```python
from build123d import *
from build123d.topology import SkipClean

# Parameters (mm, degrees)
BOSS_EXTRUDE1_DEPTH           = 3
BOSS_EXTRUDE2_START           = -1.75
SKETCH1_3_R                   = 11
BOSS_EXTRUDE2_DEPTH           = 1.75
SKETCH2_R                     = 1.75
CUT_EXTRUDE1_DEPTH            = 4.75
SKETCH2_3_R                   = 3
CUT_EXTRUDE2_DEPTH            = 1.75
SKETCH1_6_W                   = 11
SKETCH1_6_H                   = 6
BOSS_EXTRUDE3_DEPTH           = 5
SKETCH3_R                     = 1.35
CUT_EXTRUDE3_DEPTH            = 8
LPATTERN1_COUNT               = 2
LPATTERN1_PITCH               = 8
LPATTERN1_COL_COUNT           = 2
LPATTERN1_COL_PITCH           = 8
BODY_MOVE_COPY1_START         = -3
BODY_MOVE_COPY1_OUTLINE_R     = 3
BODY_MOVE_COPY1_DEPTH         = 3
BODY_MOVE_COPY1_START_2       = 3
BODY_MOVE_COPY1_2_OUTLINE_W   = 22
BODY_MOVE_COPY1_2_OUTLINE_H   = 6
BODY_MOVE_COPY1_2_OUTLINE_R   = 1.35
BODY_MOVE_COPY1_2_DEPTH       = 2
BODY_MOVE_COPY1_START_3       = 1.25
BODY_MOVE_COPY1_3_OUTLINE_R   = 3
BODY_MOVE_COPY1_3_OUTLINE_R_2 = 1.75
BODY_MOVE_COPY1_3_DEPTH       = 0.5
BODY_MOVE_COPY1_4_DEPTH       = 3
BODY_MOVE_COPY1_START_4       = 1.75
BODY_MOVE_COPY1_5_OUTLINE_R   = 11
BODY_MOVE_COPY1_5_OUTLINE_R_2 = 3
BODY_MOVE_COPY1_5_DEPTH       = 1.25
BODY_MOVE_COPY1_START_5       = -5
BODY_MOVE_COPY1_6_OUTLINE_W   = 22
BODY_MOVE_COPY1_6_OUTLINE_H   = 6
BODY_MOVE_COPY1_6_OUTLINE_R   = 1.35
BODY_MOVE_COPY1_6_DEPTH       = 2
BODY_MOVE_COPY1_START_6       = -1.75
BODY_MOVE_COPY1_7_OUTLINE_R   = 3
BODY_MOVE_COPY1_7_OUTLINE_R_2 = 1.75
BODY_MOVE_COPY1_7_DEPTH       = 0.5


# Read off the part's stored shape, not the designer's step: Body-Move/Copy1
with BuildPart() as part:
    # Sketch1 → Boss-Extrude1 (new body)
    with BuildSketch(Plane.XY):
        with BuildLine():
            Line((-11, 30), (-11, -30))
            Line((-11, -30), (11, -30))
            Line((11, -30), (11, 30))
            ThreePointArc((11, 30), (0, 41), (-11, 30))
        make_face()
        with BuildLine():
            Line((5, -23), (-5, -23))
            Line((-5, -23), (-5, 19.643842411))
            ThreePointArc((-5, 19.643842411), (0, 18.5), (5, 19.643842411))
            Line((5, 19.643842411), (5, -23))
        make_face(mode=Mode.SUBTRACT)
    extrude(amount=BOSS_EXTRUDE1_DEPTH)

    # Sketch1<3> → Boss-Extrude2 (add)
    with BuildSketch(Plane.XY.offset(BOSS_EXTRUDE2_START)):
        with Locations((0, 30)):
            Circle(SKETCH1_3_R)
    extrude(amount=BOSS_EXTRUDE2_DEPTH)

    # Sketch2 → Cut-Extrude1 (cut)
    with BuildSketch(Plane.XY.offset(3)):
        with Locations((0, 30)):
            Circle(SKETCH2_R)
    extrude(amount=-CUT_EXTRUDE1_DEPTH, mode=Mode.SUBTRACT)

    # Sketch2<3> → Cut-Extrude2 (cut)
    with BuildSketch(Plane.XY.offset(3)):
        with Locations((0, 30)):
            Circle(SKETCH2_3_R)
    extrude(amount=-CUT_EXTRUDE2_DEPTH, mode=Mode.SUBTRACT)

    # Sketch1<6> → Boss-Extrude3 (add)
    with BuildSketch(Plane.XY):
        with Locations((5.5, -27)):
            Rectangle(SKETCH1_6_W, SKETCH1_6_H)
        with Locations((-5.5, -27)):
            Rectangle(SKETCH1_6_W, SKETCH1_6_H)
    extrude(amount=-BOSS_EXTRUDE3_DEPTH)

    # Sketch3 → Cut-Extrude3 (cut)
    with BuildSketch(Plane.XY.offset(3)):
        with Locations((0, -26.6)):
            Circle(SKETCH3_R)
    cut_extrude3 = extrude(amount=-CUT_EXTRUDE3_DEPTH, mode=Mode.SUBTRACT)

    # LPattern1: Cut-Extrude3 ×2
    with Locations(*[(i * LPATTERN1_PITCH, 0, 0) for i in range(1, LPATTERN1_COUNT)]):
        add(cut_extrude3, mode=Mode.SUBTRACT)

    # LPattern1 col: Cut-Extrude3 ×2
    with Locations(*[(-i * LPATTERN1_COL_PITCH, 0, 0) for i in range(1, LPATTERN1_COL_COUNT)]):
        add(cut_extrude3, mode=Mode.SUBTRACT)

    # Body-Move/Copy1 outline → Body-Move/Copy1 (add)
    with BuildSketch(Plane.XY.offset(BODY_MOVE_COPY1_START)):
        with BuildLine():
            Line((-11, 30), (-11, -24))
            Line((-11, -24), (11, -24))
            Line((11, -24), (11, 30))
            ThreePointArc((11, 30), (0, 41), (-11, 30))
        make_face()
        with BuildLine():
            Line((-5, -23), (-5, 19.643842411))
            ThreePointArc((-5, 19.643842411), (0, 18.5), (5, 19.643842411))
            Line((5, 19.643842411), (5, -23))
            Line((5, -23), (-5, -23))
        make_face(mode=Mode.SUBTRACT)
        with Locations((0, 30)):
            Circle(BODY_MOVE_COPY1_OUTLINE_R, mode=Mode.SUBTRACT)
    extrude(amount=BODY_MOVE_COPY1_DEPTH)

    # Body-Move_Copy1 2 outline → Body-Move_Copy1 2 (add)
    with BuildSketch(Plane.XY.offset(BODY_MOVE_COPY1_START_2)):
        with Locations((0, -27)):
            Rectangle(BODY_MOVE_COPY1_2_OUTLINE_W, BODY_MOVE_COPY1_2_OUTLINE_H)
        with Locations((-8, -26.6)):
            Circle(BODY_MOVE_COPY1_2_OUTLINE_R, mode=Mode.SUBTRACT)
        with Locations((0, -26.6)):
            Circle(BODY_MOVE_COPY1_2_OUTLINE_R, mode=Mode.SUBTRACT)
        with Locations((8, -26.6)):
            Circle(BODY_MOVE_COPY1_2_OUTLINE_R, mode=Mode.SUBTRACT)
    extrude(amount=BODY_MOVE_COPY1_2_DEPTH)

    # Body-Move_Copy1 3 outline → Body-Move_Copy1 3 (add)
    with BuildSketch(Plane.XY.offset(BODY_MOVE_COPY1_START_3)):
        with Locations((0, 30)):
            Circle(BODY_MOVE_COPY1_3_OUTLINE_R)
        with Locations((0, 30)):
            Circle(BODY_MOVE_COPY1_3_OUTLINE_R_2, mode=Mode.SUBTRACT)
    extrude(amount=BODY_MOVE_COPY1_3_DEPTH)

    # Body-Move_Copy1 4 outline → Body-Move_Copy1 4 (cut)
    with SkipClean():  # the faces are left unmerged after this step: merging them gives an invalid solid
        with BuildSketch(Plane.XY):
            with BuildLine():
                Line((-11, 30), (-11, -24))
                Line((-11, -24), (11, -24))
                Line((11, -24), (11, 30))
                ThreePointArc((11, 30), (0, 19), (-11, 30))
            make_face()
            with BuildLine():
                Line((-5, -23), (-5, 19.643842411))
                ThreePointArc((-5, 19.643842411), (0, 18.5), (5, 19.643842411))
                Line((5, 19.643842411), (5, -23))
                Line((5, -23), (-5, -23))
            make_face(mode=Mode.SUBTRACT)
        extrude(amount=BODY_MOVE_COPY1_4_DEPTH, mode=Mode.SUBTRACT)

    # Body-Move_Copy1 5 outline → Body-Move_Copy1 5 (cut)
    with BuildSketch(Plane.XY.offset(BODY_MOVE_COPY1_START_4)):
        with Locations((0, 30)):
            Circle(BODY_MOVE_COPY1_5_OUTLINE_R)
        with Locations((0, 30)):
            Circle(BODY_MOVE_COPY1_5_OUTLINE_R_2, mode=Mode.SUBTRACT)
    extrude(amount=BODY_MOVE_COPY1_5_DEPTH, mode=Mode.SUBTRACT)

    # Body-Move_Copy1 6 outline → Body-Move_Copy1 6 (cut)
    with BuildSketch(Plane.XY.offset(BODY_MOVE_COPY1_START_5)):
        with Locations((0, -27)):
            Rectangle(BODY_MOVE_COPY1_6_OUTLINE_W, BODY_MOVE_COPY1_6_OUTLINE_H)
        with Locations((-8, -26.6)):
            Circle(BODY_MOVE_COPY1_6_OUTLINE_R, mode=Mode.SUBTRACT)
        with Locations((0, -26.6)):
            Circle(BODY_MOVE_COPY1_6_OUTLINE_R, mode=Mode.SUBTRACT)
        with Locations((8, -26.6)):
            Circle(BODY_MOVE_COPY1_6_OUTLINE_R, mode=Mode.SUBTRACT)
    extrude(amount=BODY_MOVE_COPY1_6_DEPTH, mode=Mode.SUBTRACT)

    # Body-Move_Copy1 7 outline → Body-Move_Copy1 7 (cut)
    with BuildSketch(Plane.XY.offset(BODY_MOVE_COPY1_START_6)):
        with Locations((0, 30)):
            Circle(BODY_MOVE_COPY1_7_OUTLINE_R)
        with Locations((0, 30)):
            Circle(BODY_MOVE_COPY1_7_OUTLINE_R_2, mode=Mode.SUBTRACT)
    extrude(amount=BODY_MOVE_COPY1_7_DEPTH, mode=Mode.SUBTRACT)


solid = part.part
```
Work out the finished part from the listing and answer in its coordinate system (mm). A direction names the side the tool comes from. Give positions to 0.01 mm unless a question says otherwise; leave off trailing zeros. Write each loop counter-clockwise with the first axis right and the second up, starting at its lowest first coordinate (ties: lowest second). Pieces come first, ordered by that corner, then holes.
(1) Which of the six approach directions +Z, -Z, +X, -X, +Y, -Y give full straight-line access (tool end or side, diameter ignored) to faces 4 (the flat face through (5, -1, -2)), 5 (the flat face through (0, 28, -1.25))?
Final values:
face 4: +Z, -Z
face 5: -Z
(2) Flat-ended cylindrical pins translate along their axes: pin 1 Ø1.6 at (x, y) = (-8, -26.6) entering from -Z; pin 2 Ø3 at (x, y) = (-0.5, 31) entering from +Z; pin 3 Ø6 at (x, y) = (-3, -1.5) entering from +Z; pin 4 Ø1 at (x, z) = (-7.5, 0) entering from +Y. Find the tip coordinate at first contact, or state that the pin passes through.
Final values:
pin 1: passes through
pin 2: stops at z = 1.75
pin 3: stops at z = 0
pin 4: stops at y = 38.49
(3) Straight lines are drawn through the part: line 1 (Y direction, x = 0, z = -0.35); line 2 (X direction, y = 0, z = -2.5); line 3 (Y direction, x = 0, z = 4.5). For each, find the intervals that lie inside material, in ascending order.
Final values:
line 1: y = -30 to -27.95, -25.25 to -23, 18.5 to 28.25, 31.75 to 41
line 2: x = -11 to -5, 5 to 11
line 3: y = -30 to -27.95, -25.25 to -24
(4) The part is cut by section A-A on x = 0. Write down the section's boundary in (y, z).
Final values:
outline: (-30, -3) - (-27.95, -3) - (-27.95, 5) - (-30, 5) - close; (-25.25, -3) - (-23, -3) - (-23, 0) - (-24, 0) - (-24, 5) - (-25.25, 5) - close; (18.5, -3) - (27, -3) - (27, -1.25) - (28.25, -1.25) - (28.25, 1.75) - (19, 1.75) - (19, 0) - (18.5, 0) - close; (31.75, -1.25) - (33, -1.25) - (33, -3) - (41, -3) - (41, 1.75) - (31.75, 1.75) - close
(5) The part is cut by section B-B on y = -11. Write down the section's boundary in (x, z).
Final values:
outline: (-11, -3) - (-5, -3) - (-5, 0) - (-11, 0) - close; (5, -3) - (11, -3) - (11, 0) - (5, 0) - close
(6) The mould has two halves that part along Y. Classify faces 1 (the flat face through (0, -23, -2)), 2 (the flat face through (-5, -2, -2)), 3 (the flat face through (-0.2, -28.3, 5)): pulls with the +Y half, pulls with the -Y half, needs draft (parallel to the pull), parting line crosses it, or undercut.
Final values:
face 1: undercut
face 2: undercut
face 3: needs draft
(7) The part is cut by section C-C on z = 4. Write down the section's boundary in (x, y), plus the area to 3 significant figures.
Final values:
outline: (-11, -30) - (11, -30) - (11, -24) - (-11, -24) - close; hole circle Ø2.7 at (-8, -26.6); hole circle Ø2.7 at (0, -26.6); hole circle Ø2.7 at (8, -26.6)
area: 115 mm2
(8) The part is cut by section D-D on x = -4. Write down the section's boundary in (y, z), plus the area to 3 significant figures.
Final values:
outline: (-30, -3) - (-23, -3) - (-23, 0) - (-24, 0) - (-24, 5) - (-30, 5) - close; (19.22, -3) - (40.25, -3) - (40.25, 1.75) - (19.75, 1.75) - (19.75, 0) - (19.22, 0) - close
area: 150 mm2
